Verification items for the finished model (mm, model axes). A direction names the side the tool comes from. Round coordinates to 2 decimals unless told otherwise and drop trailing zeros. Write each loop counter-clockwise with the first axis right and the second up, starting at its lowest first coordinate (ties: lowest second). Pieces come first, ordered by that corner, then holes. Notation, with made-up numbers: (67.5, 45.25) -> (95.5, 45.25) arc R18 cw to (95.5, 58.25) -> close; hole circle Ø8 at (-33, 72). An arc over 180 degrees is marked (long way). Use CSV: the item, a comma, the result in double quotes.
```python
from build123d import *

# Parameters (mm, degrees)
X_GUIDE_EXTRUDE_DEPTH   = 279.4
END_PLATE_HOLES_D       = 4.0386
END_PLATE_HOLES_DEPTH   = 11.938
END_PLATE_HOLES_TIP     = 1.213317848
END_PLATE_HOLES_2_D     = 4.0386
END_PLATE_HOLES_2_DEPTH = 11.938
END_PLATE_HOLES_2_TIP   = 1.213317848


with BuildPart() as part:
    # dovetail-male-profile → x-guide-extrude (new body)
    with BuildSketch(Plane.XY):
        Polygon((47.331706063, 31.242), (16.383, 31.242), (16.383, 12.192), (-16.383, 12.192), (-16.383, 31.242), (-39.999357645, 31.242), (-31.127216058, 15.875), (-63.5, 15.875), (-63.5, 0), (63.5, 0), (63.5, 15.875), (38.459564477, 15.875), align=None)
    extrude(amount=X_GUIDE_EXTRUDE_DEPTH)

    # end plate holes
    with Locations(Plane(origin=(0, 0, 0), x_dir=(-1, 0, 0), z_dir=(0, 0, -1))):
        with Locations((-25.4, 23.8125), (25.4, 23.8125), (25.4, 7.874), (-25.4, 7.874)):
            Hole(END_PLATE_HOLES_D / 2, depth=END_PLATE_HOLES_DEPTH)
            with Locations((0, 0, -(END_PLATE_HOLES_DEPTH + END_PLATE_HOLES_TIP / 2))):  # 118° drill point
                Cone(0, END_PLATE_HOLES_D / 2, END_PLATE_HOLES_TIP, mode=Mode.SUBTRACT)

    # end plate holes 2
    with Locations(Plane.XY.offset(279.4)):
        with Locations((25.4, 23.8125), (25.4, 7.874), (-25.4, 7.874), (-25.4, 23.8125)):
            Hole(END_PLATE_HOLES_2_D / 2, depth=END_PLATE_HOLES_2_DEPTH)
            with Locations((0, 0, -(END_PLATE_HOLES_2_DEPTH + END_PLATE_HOLES_2_TIP / 2))):  # 118° drill point
                Cone(0, END_PLATE_HOLES_2_D / 2, END_PLATE_HOLES_2_TIP, mode=Mode.SUBTRACT)


solid = part.part
```
Q1. Material ranges on L1, parallel to Y at x = -25.4, z = 9.75; L2, parallel to X at y = 15.5, z = 180; L3, parallel to Y at x = -56.5, z = 85 (3 decimals), recorded low to high.
Filled in:
L1,"0 to 5.85, 9.89 to 21.79, 25.83 to 31.24"
L2,"-63.5 to -16.38, 16.38 to 63.5"
L3,"0 to 15.875"
Q2. Access from +Z, -Z, +X, -X, +Y, -Y to the whole of each face (thin tool, end or side, straight path). Record for faces 1 (the flat face through (-47, 15.875, 138)), 2 (the flat face through (-16.383, 22, 138)), 3 (the flat face through (32, 31.242, 138)), 4 (the flat face through (63.5, 8, 138)), 5 (the flat face through (42.834, 23.451, 137.744)).
Filled in:
face 1,"+Z, -Z, -X"
face 2,"+Z, -Z, +Y"
face 3,"+Z, -Z, +X, -X, +Y"
face 4,"+Z, -Z, +X, +Y, -Y"
face 5,"+Z, -Z, +X"
Q3. Section check A-A (z = 28.5). Record the cut outline in (x, y) (3 decimals), plus the area to 3 significant figures.
Filled in:
outline,"(-63.5, 0) -> (63.5, 0) -> (63.5, 15.875) -> (38.46, 15.875) -> (47.332, 31.242) -> (16.383, 31.242) -> (16.383, 12.192) -> (-16.383, 12.192) -> (-16.383, 31.242) -> (-39.999, 31.242) -> (-31.127, 15.875) -> (-63.5, 15.875) -> close"
area,"2,600 mm²"
Q4. Section check B-B (x = -36). Record the cut outline in (y, z) (3 decimals).
Filled in:
outline,"(0, 0) -> (15.875, 0) -> (15.875, 279.4) -> (0, 279.4) -> close; (24.315, 0) -> (31.242, 0) -> (31.242, 279.4) -> (24.315, 279.4) -> close"
Q5. Go/stop test with flat-tipped pins: P1, Ø2.5, axis at x = 25.4, y = 23.81, coming from the -Z side; P2, Ø1.5, axis at y = 25, z = 75.5, coming from the +X side; P3, Ø2.5, axis at x = 25.4, y = 23.81, coming from the +Z side. Record where each tip stops, or that it passes through.
Filled in:
P1,"z = 12.4"
P2,"x = 44.16"
P3,"z = 267"
Q6. Section check D-D (x = -1). Record the cut outline in (y, z).
Filled in:
outline,"(0, 0) -> (12.19, 0) -> (12.19, 279.4) -> (0, 279.4) -> close"
Q7. Mould release check, pull along X, two halves, no side actions. Record for faces 6 (the flat face through (-35.625, 23.666, 137.744)), 7 (the flat face through (0, 12.192, 138)), 8 (the flat face through (16.383, 22, 138)), 9 (the flat face through (-28, 31.242, 138)): released by +X, released by -X, zero draft, split by the parting line, or undercut.
Filled in:
face 6,"released by -X"
face 7,"undercut"
face 8,"undercut"
face 9,"zero draft"
Q8. Section check C-C (x = 52). Record the cut outline in (y, z) (3 decimals).
Filled in:
outline,"(0, 0) -> (15.875, 0) -> (15.875, 279.4) -> (0, 279.4) -> close"
